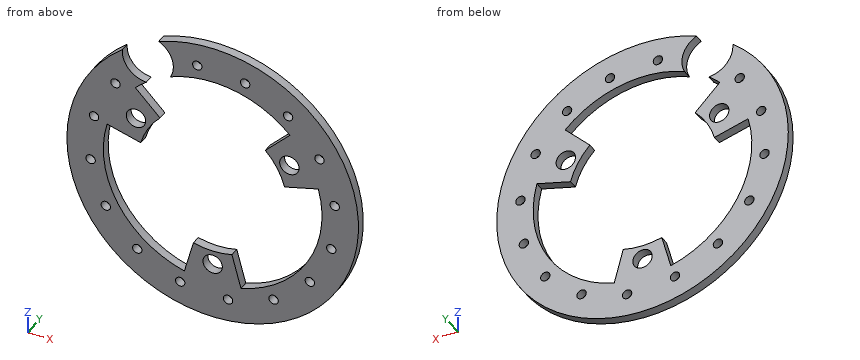
from build123d import *

# Parameters (mm, degrees)
SKETCH1_R          = 101.6
EXTRUDE1_DEPTH     = 6.35
SKETCH3_R          = 51.8922
CUT_EXTRUDE2_DEPTH = 6.35
SKETCH5_R          = 6.746875
CUT_EXTRUDE4_DEPTH = 6.35
CIRPATTERN1_COUNT  = 3
SKETCH16_R         = 17.78
CUT_EXTRUDE5_DEPTH = 6.35
CUT_EXTRUDE9_DEPTH = 6.35
CIRPATTERN2_COUNT  = 3
CIRPATTERN3_COUNT  = 16


with BuildPart() as part:
    # Sketch1 → Extrude1 (new body)
    with BuildSketch(Plane(origin=(0, 0, 0), x_dir=(1, 0, 0), z_dir=(0, 1, 0))):
        with Locations(Location((0, 0, 0), (0, 0, 270))):
            Circle(SKETCH1_R)
    extrude(amount=EXTRUDE1_DEPTH)

    # Sketch3 → Cut-Extrude2 (cut)
    with BuildSketch(Plane(origin=(0, 0, 0), x_dir=(1, 0, 0), z_dir=(0, 1, 0))):
        with Locations(Location((0, 0, 0), (0, 0, 270))):
            Circle(SKETCH3_R)
    extrude(amount=CUT_EXTRUDE2_DEPTH, mode=Mode.SUBTRACT)

    # Sketch5 → Cut-Extrude4 (cut)
    with BuildSketch(Plane(origin=(0, 0, 0), x_dir=(1, 0, 0), z_dir=(0, 1, 0))):
        with Locations(Location((0, 61.722, 0), (0, 0, 270))):
            Circle(SKETCH5_R)
    cut_extrude4 = extrude(amount=CUT_EXTRUDE4_DEPTH, mode=Mode.SUBTRACT)

    # CirPattern1: Cut-Extrude4 ×3 about axis
    cirpattern1_axis = Axis((0, 0, 0), (0, 1, 0))
    for i in range(1, CIRPATTERN1_COUNT):
        add(cut_extrude4.rotate(cirpattern1_axis, i * 360 / CIRPATTERN1_COUNT), mode=Mode.SUBTRACT)

    # Sketch16 → Cut-Extrude5 (cut)
    with BuildSketch(Plane(origin=(0, 0, 0), x_dir=(1, 0, 0), z_dir=(0, 1, 0))):
        with Locations((-45.212, -78.309481112)):
            Circle(SKETCH16_R)
    extrude(amount=CUT_EXTRUDE5_DEPTH, mode=Mode.SUBTRACT)

    # Sketch17 → Cut-Extrude9 (cut)
    with BuildSketch(Plane(origin=(0, 0, 0), x_dir=(1, 0, 0), z_dir=(0, 1, 0))):
        with BuildLine():
            Line((-13.430689652, 50.124016163), (-19.722011237, 73.603547963))
            ThreePointArc((-19.722011237, 73.603547963), (-65.991135768, 38.1), (-73.603547963, -19.722011237))
            Line((-73.603547963, -19.722011237), (-50.124016163, -13.430689652))
            ThreePointArc((-50.124016163, -13.430689652), (-44.939963458, 25.9461), (-13.430689652, 50.124016163))
        make_face()
    cut_extrude9 = extrude(amount=CUT_EXTRUDE9_DEPTH, mode=Mode.SUBTRACT)

    # CirPattern2: Cut-Extrude9 ×3 about axis
    cirpattern2_axis = Axis((0, 0, 0), (0, 1, 0))
    for i in range(1, CIRPATTERN2_COUNT):
        add(cut_extrude9.rotate(cirpattern2_axis, i * 360 / CIRPATTERN2_COUNT), mode=Mode.SUBTRACT)

    # Sketch23 → F (0.257) Diameter Hole1 (revolve, cut)
    with BuildSketch(Plane(origin=(42.459430359, 6.35, -74.471285732), x_dir=(0, 0, 1), z_dir=(1, 0, 0))):
        Polygon((0, 0), (0, 60.381148974), (3.2639, 58.42), (3.2639, 0), align=None)
    f_0_257_diameter_hole1 = revolve(axis=Axis((42.459430359, 12.7, -74.471285732), (0, -1, 0)), mode=Mode.SUBTRACT)

    # CirPattern3: F (0.257) Diameter Hole1 ×16 about axis, 1 skipped
    cirpattern3_axis = Axis((0, 0, 0), (0, 1, 0))
    add([f_0_257_diameter_hole1.rotate(cirpattern3_axis, i * 360 / CIRPATTERN3_COUNT) for i in range(1, CIRPATTERN3_COUNT) if i not in (8,)], mode=Mode.SUBTRACT)


solid = part.part
Could you check a few things on this model? Use its own coordinates, in mm. Give positions to 0.01 mm unless a question says otherwise; leave off trailing zeros. Loops run counter-clockwise (first coordinate to the right, second up) from the corner with the lowest first, then second, coordinate; pieces in that order, holes last. Notation, with made-up numbers: M 33,29 L 43,29 A8 ccw 43,38 Z; hole C 88.25,14.25 d8. An arc over 180 degrees is marked long. Answer as a JSON object with one key per item and string values.
Q1. Suppose I cut it at B-B, the plane x = 0. List the corners of the cut face in (y, z) for me.
Values found:
{"outline": "M 0,-101.6 L 6.35,-101.6 L 6.35,-68.47 L 0,-68.47 Z; M 0,-54.98 L 6.35,-54.98 L 6.35,-51.89 L 0,-51.89 Z; M 0,76.2 L 6.35,76.2 L 6.35,101.6 L 0,101.6 Z"}
Q2. If I drill on probe 1 along X at (y, z) = (3, -20.5); probe 2 along Z at (x, y) = (-70, 3.25); probe 3 along Z at (x, y) = (-57.5, 6), over which ranges is the centre line in solid material (lowest first)? Write a range as [from, to].
Values found:
{"probe 1": "x = [-99.51, -73.39], [73.39, 80.21], [85.15, 99.51]", "probe 2": "z = [-73.64, -30.11], [18.76, 50.21], [54.9, 73.64]", "probe 3": "z = [-83.76, -50], [15.41, 25.46], [36.26, 65.46]"}
Q3. Suppose I cut it at C-C, the plane x = 32.5. List the corners of the cut face in (y, z) for me, plus the area to 3 significant figures.
Values found:
{"outline": "M 0,-96.26 L 6.35,-96.26 L 6.35,-68.92 L 0,-68.92 Z; M 0,68.92 L 6.35,68.92 L 6.35,96.26 L 0,96.26 Z", "area": "347 mm²"}
Q4. For P1, Ø1.5, axis at x = 50, y = 4.5, coming from the +Z side; P2, Ø4, axis at x = -74.47, z = -42.46, coming from the -Y side; P3, Ø1, axis at y = 1, z = -65.5, coming from the -X side; P4, Ø3, axis at y = 1, z = -61, coming from the +X side, each with a flat end and sliding along its axis, tell me the tip position at first contact or that it passes through.
Values found:
{"P1": "stops at z = 88.87", "P2": "passes through", "P3": "stops at x = -78.09", "P4": "stops at x = 82.35"}
Q5. Suppose I cut it at D-D, the plane y = 1.25. State how many separate pieces and enclosed holes the cut face has, plus the area to 3 significant figures.
Values found:
{"separate pieces": "1", "enclosed holes": "18", "area": "14,900 mm²"}
Q6. Suppose I cut it at A-A, the plane z = 0. List the corners of the cut face in (x, y) for me, plus the area to 3 significant figures.
Values found:
{"outline": "M -101.6,0 L -76.2,0 L -76.2,6.35 L -101.6,6.35 Z; M 76.2,0 L 101.6,0 L 101.6,6.35 L 76.2,6.35 Z", "area": "323 mm²"}
